Read the model definition and answer for the solid it produces. Units are mm, in the model's axes. A direction names the side the tool comes from. Give positions to 0.01 mm unless a question says otherwise; leave off trailing zeros. Order: outer loops, then holes, each group sorted by start corner. A loop starts at its lowest first (then second) coordinate and runs counter-clockwise, first axis right, second up. Notation, with made-up numbers: (73.5, 22.25) - (82.5, 22.25) arc R24 cw to (82.5, 44.25) - close; hole circle Ø8 at (87, -6). An arc over 180 degrees is marked (long way). Use a Markdown table: item, result. Add a question column.
1. Flat-ended cylindrical pins translate along their axes: P1, Ø0.6, axis at y = -6, z = 2.5, coming from the +X side; P2, Ø1.5, axis at y = -1, z = 2.5, coming from the -X side; P3, Ø1.3, axis at y = 5.5, z = 2, coming from the +X side; P4, Ø4, axis at x = 7, y = -14, coming from the +Z side. Find the tip coordinate at first contact, or state that the pin passes through.
2. A cutting plane is placed at B-B on y = -14. State how many separate pieces and enclosed holes the cut face has, and give its area (3 significant figures).
3. A cutting plane is placed at A-A on x = 0. Determine the outline of the cut face in (y, z) (3 decimals), and give its area (3 significant figures).
4. Consider L1, parallel to X at y = -12, z = 0.2; L2, parallel to Z at x = -4.5, y = 5; L3, parallel to Y at x = 5.5, z = 1.15. Determine where each line is inside the solid, lowest interval first.
5. Which of the six approach directions +Z, -Z, +X, -X, +Y, -Y give full straight-line access (tool end or side, diameter ignored) to faces 5 (the cylindrical face through (8.166, -0.014, 2.092)), 6 (the cylindrical face through (4.225, 0.014, 2.092)), 7 (the flat face through (1, -6, 2))?
6. For a pull along X with two mould halves and no side action, classify faces 1 (the flat face through (-1, 6, 2)), 2 (the flat face through (0, 6, 3)), 3 (the flat face through (1, 6, 2)), 4 (the cylindrical face through (-8.15, -11.78, 0.76)) as released by +X, released by -X, zero draft, split by the parting line, or undercut.
```python
from build123d import *

# Parameters (mm, degrees)
F0_R     = 20
F1_DEPTH = 1.5
F2_D     = 5
F2_DEPTH = 20.381
F2_TIP   = 1.5021515476
F3_R     = 2
F4_DEPTH = 3
F5_SIZE  = 0.3


# Not quite as in the source:
# - a pattern or mirror of a feature is missing from the dataset's text; its kind, count and spacing are read off the source's solid


with BuildPart() as f1:
    # F0 (on Top) → F1 (new body)
    with BuildSketch(Plane.XY):
        Circle(F0_R)
    extrude(amount=F1_DEPTH)

    # F2
    with Locations(Plane(origin=(0, 0, 0), x_dir=(1, 0, 0), z_dir=(0, 0, -1))):
        with Locations((-7, 14)):
            f2 = Hole(F2_D / 2, depth=F2_DEPTH)
            with Locations((0, 0, -(F2_DEPTH + F2_TIP / 2))):  # 118° drill point
                Cone(0, F2_D / 2, F2_TIP, mode=Mode.SUBTRACT)

    # F2_copies: F2 across plane
    add(f2.mirror(Plane(origin=(0, 0, 0), x_dir=(0, 0, 1), z_dir=(1, 0, 0))), mode=Mode.SUBTRACT)

    # F3 (on Top) → F4 (join)
    with BuildSketch(Plane.XY):
        with BuildLine():
            Line((-4.104842454, 1.0004466142), (-8.104842454, 1.0004466142))
            ThreePointArc((-8.104842454, 1.0004466142), (-8.1663556518, 0), (-8.104842454, -1.0004466142))
            Line((-8.104842454, -1.0004466142), (-4.104842454, -1.0004466142))
            ThreePointArc((-4.104842454, -1.0004466142), (-4.225, 0), (-4.104842454, 1.0004466142))
        make_face()
        with BuildLine():
            ThreePointArc((1, 8.1048975707), (0, 8.1663556518), (-1, 8.1048975707))
            Line((-1, 8.1048975707), (-1, 4.1049512786))
            ThreePointArc((-1, 4.1049512786), (0, 4.225), (1, 4.1049512786))
            Line((1, 4.1049512786), (1, 8.1048975707))
        make_face()
        with BuildLine():
            Line((4.104842454, -1.0004466142), (8.104842454, -1.0004466142))
            ThreePointArc((8.104842454, -1.0004466142), (8.1663556518, 0), (8.104842454, 1.0004466142))
            Line((8.104842454, 1.0004466142), (4.104842454, 1.0004466142))
            ThreePointArc((4.104842454, 1.0004466142), (4.225, 0), (4.104842454, -1.0004466142))
        make_face()
        with BuildLine():
            ThreePointArc((-1, -8.1048975707), (0, -8.1663556518), (1, -8.1048975707))
            Line((1, -8.1048975707), (1, -4.1049512786))
            ThreePointArc((1, -4.1049512786), (0, -4.225), (-1, -4.1049512786))
            Line((-1, -4.1049512786), (-1, -8.1048975707))
        make_face()
        Circle(F3_R)
    extrude(amount=F4_DEPTH)

    # F5
    f5_edges = [f1.edges().sort_by_distance(p)[0] for p in [
        (-2, 0, 3),
        (0, 8.166356, 3),
        (-1, 6.104924, 3),
        (0, 4.225, 3),
        (1, 6.104924, 3),
        (6.104842, -1.000447, 3),
        (8.166356, 0, 3),
        (6.104842, 1.000447, 3),
        (4.225, 0, 3),
        (1, -6.104924, 3),
        (0, -4.225, 3),
        (-1, -6.104924, 3),
        (0, -8.166356, 3),
        (-6.104842, 1.000447, 3),
        (-8.166356, 0, 3),
        (-6.104842, -1.000447, 3),
        (-4.225, 0, 3),
        (-20, 0, 1.5),
    ]]
    chamfer(f5_edges, length=F5_SIZE)


solid = f1.part
```
Output values:
| question | item | result |
|---|---|---|
| 1 | P1 | x = 1 |
| 1 | P2 | x = -8.16 |
| 1 | P3 | x = 19.1 |
| 1 | P4 | through |
| 2 | separate pieces | 3 |
| 2 | enclosed holes | 0 |
| 2 | area | 27.7 mm² |
| 3 | outline | (-20, 0) - (20, 0) - (20, 1.2) - (19.7, 1.5) - (8.166, 1.5) - (8.166, 2.7) - (7.866, 3) - (4.525, 3) - (4.225, 2.7) - (4.225, 1.5) - (2, 1.5) - (2, 2.7) - (1.7, 3) - (-1.7, 3) - (-2, 2.7) - (-2, 1.5) - (-4.225, 1.5) - (-4.225, 2.7) - (-4.525, 3) - (-7.866, 3) - (-8.166, 2.7) - (-8.166, 1.5) - (-19.7, 1.5) - (-20, 1.2) - close |
| 3 | area | 77.5 mm² |
| 4 | L1 | -16 to -8.5, -5.5 to 5.5, 8.5 to 16 |
| 4 | L2 | 0 to 1.5 |
| 4 | L3 | -19.23 to -16, -12 to 19.23 |
| 5 | face 5 | +Z, +X |
| 5 | face 6 | +Z |
| 5 | face 7 | +Z, +X, -Y |
| 6 | face 1 | released by -X |
| 6 | face 2 | zero draft |
| 6 | face 3 | released by +X |
| 6 | face 4 | undercut |
